Geometry check sheet. Reference: the model listing, model coordinates, mm. Face numbers are marked on the shaded views. Coordinates: 2 decimals unless noted, no trailing zeros. Loops run counter-clockwise (first coordinate to the right, second up) from the corner with the lowest first, then second, coordinate; pieces in that order, holes last.
from build123d import *

# Parameters (mm, degrees)
CYLINDER233_R          = 3.2
CYLINDER233_DEPTH      = 16
CYLINDER_R             = 5
CYLINDER_DEPTH         = 4.5
CUT277_PLACEMENT_ANGLE = 90


with BuildPart() as cylinder233:
    # Cylinder233 → Cylinder233 (new body)
    with BuildSketch(Plane.XY.offset(-3)):
        Circle(CYLINDER233_R)
    extrude(amount=CYLINDER233_DEPTH)


with BuildPart() as cut277:
    # Cylinder → Cylinder (new body)
    with BuildSketch(Plane.XY):
        Circle(CYLINDER_R)
    extrude(amount=CYLINDER_DEPTH)

    # Cut277: cut Cylinder233
    add(cylinder233.part, mode=Mode.SUBTRACT)


with BuildPart() as cut277_1:
    # Cut277 placement: moved
    add(cut277.part.moved(Location((114, -3.3, 62.4))).rotate(Axis((114, -3.3, 62.4), (1, 0, 0)), CUT277_PLACEMENT_ANGLE))


solid = cut277_1.part
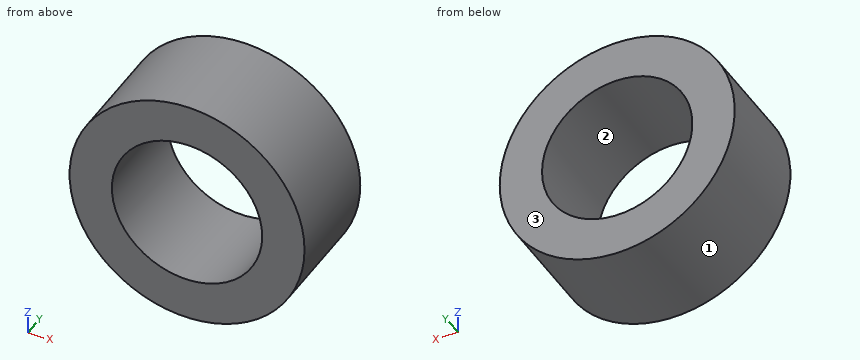
(1) Sectioned sample at C-C on y = -5.1. Record the cut outline in (x, z).
Findings:
outline: circle Ø10 at (114, 62.4); hole circle Ø6.4 at (114, 62.4)
(2) Sectioned sample at D-D on x = 118. Record the cut outline in (y, z), and give its area (3 significant figures).
Findings:
outline: (-7.8, 59.4) - (-3.3, 59.4) - (-3.3, 65.4) - (-7.8, 65.4) - close
area: 27.0 mm2
(3) Gauge pin test, flat ends, axial feed: pin 1 Ø5 at (x, z) = (116, 64.5) entering from +Y; pin 2 Ø3 at (x, z) = (115.5, 62) entering from -Y. Record the tip position at first contact, or that the pin passes through.
Findings:
pin 1: stops at y = -3.3
pin 2: passes through
(4) Scan lines: L1, parallel to Z at x = 114, y = -6.15; L2, parallel to X at y = -4.65, z = 64.5; L3, parallel to X at y = -6.4, z = 59.75. Record each from-to range of solid material in increasing order.
Findings:
L1: z = 57.4 to 59.2, 65.6 to 67.4
L2: x = 109.46 to 111.59, 116.41 to 118.54
L3: x = 109.76 to 112.21, 115.79 to 118.24
(5) Draft check along X on the marked faces 1, 2 and 3. Enter one of: +X half, -X half, draft (parallel to the pull), parting line (faces both ways), or undercut.
Findings:
face 1: parting line
face 2: undercut
face 3: draft
(6) Sectioned sample at A-A on z = 62.4. Record the cut outline in (x, y), and give its area (3 significant figures).
Findings:
outline: (109, -7.8) - (110.8, -7.8) - (110.8, -3.3) - (109, -3.3) - close; (117.2, -7.8) - (119, -7.8) - (119, -3.3) - (117.2, -3.3) - close
area: 16.2 mm2
(7) Sectioned sample at B-B on x = 114. Record the cut outline in (y, z), and give its area (3 significant figures).
Findings:
outline: (-7.8, 57.4) - (-3.3, 57.4) - (-3.3, 59.2) - (-7.8, 59.2) - close; (-7.8, 65.6) - (-3.3, 65.6) - (-3.3, 67.4) - (-7.8, 67.4) - close
area: 16.2 mm2
